The figure shows three views and two pictorial views of one solid part (mm, origin at its lowest corner). Answer the questions. Round coordinates to 2 decimals unless told otherwise and drop trailing zeros. Write each loop counter-clockwise with the first axis right and the second up, starting at its lowest first coordinate (ties: lowest second). Pieces come first, ordered by that corner, then holes. Notation, with made-up numbers: M 56.25,53 L 64.25,53 A10 ccw 64.25,72 Z; hole C 42.25,-8 d3. An arc over 180 degrees is marked long. Answer in a Markdown table with one row per item.
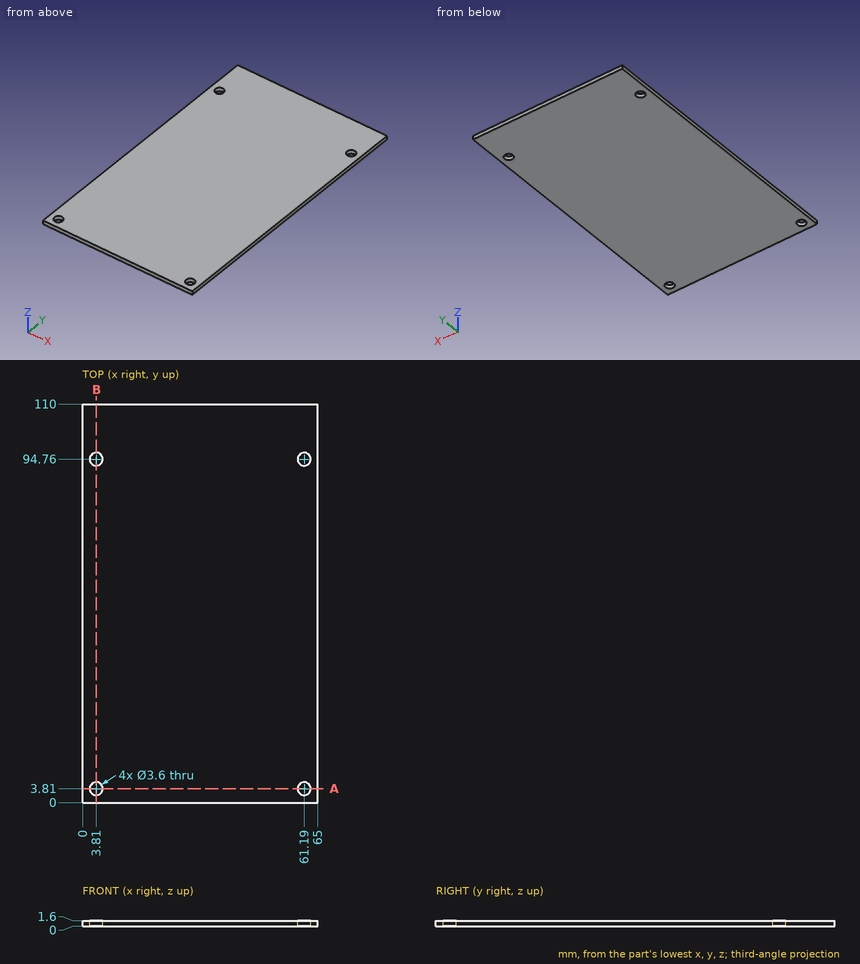
1. The part is cut by section B-B (x = 3.81). Determine the outline of the cut face in (y, z), plus the area to 3 significant figures.
Calculated:
| item | result |
|---|---|
| outline | M 0,0 L 2.01,0 L 2.01,1.6 L 0,1.6 Z; M 5.61,0 L 92.96,0 L 92.96,1.6 L 5.61,1.6 Z; M 96.56,0 L 110,0 L 110,1.6 L 96.56,1.6 Z |
| area | 164 mm² |
2. The part is cut by section A-A (y = 3.81). Determine the outline of the cut face in (x, z), plus the area to 3 significant figures.
Calculated:
| item | result |
|---|---|
| outline | M 0,0 L 2.01,0 L 2.01,1.6 L 0,1.6 Z; M 5.61,0 L 59.39,0 L 59.39,1.6 L 5.61,1.6 Z; M 62.99,0 L 65,0 L 65,1.6 L 62.99,1.6 Z |
| area | 92.5 mm² |
3. Consider line 1 along X through (y, z) = (94.76, 1.15); line 2 along Y through (x, z) = (3.81, 1.1). Determine where each line is inside the solid, lowest interval first. Write a range as from..to.
Calculated:
| item | result |
|---|---|
| line 1 | x = 0..2.01, 5.61..59.39, 62.99..65 |
| line 2 | y = 0..2.01, 5.61..92.96, 96.56..110 |
4. Given pin 1 (6 mm diameter, centred on x = 11, y = 61.5, fed in from -Z); pin 2 (3 mm diameter, centred on x = 3.81, y = 3.81, fed in from +Z), each flat-ended and moving along its own axis, determine where each tip first touches the part or whether it passes through.
Calculated:
| item | result |
|---|---|
| pin 1 | stops at z = 0 |
| pin 2 | passes through |
